```python
from build123d import *

# Parameters (mm, degrees)
F0_R     = 43.18
F1_DEPTH = 330.2
F3_DEPTH = 71.12
F4_R     = 19.05
F5_DEPTH = 76.2
F6_R     = 165.1
F6_R_2   = 19.05
F7_DEPTH = 50.8
F8_R     = 25.39999


# Not quite as in the source:
# - a fillet or chamfer is up to 0.001 mm smaller than in the source, because OpenCascade refuses the exact size


with BuildPart() as f1:
    # F0 (on Top) → F1 (new body)
    with BuildSketch(Plane.XY):
        Circle(F0_R)
    extrude(amount=F1_DEPTH)

    # F2 (on face) → F3 (cut)
    with BuildSketch(Plane(origin=(0, 0, 0), x_dir=(1, 0, 0), z_dir=(0, 0, -1))):
        with BuildLine():
            ThreePointArc((43.18, 0), (40.8909417637, 13.8723927885), (34.2664621733, 26.2739789549))
            Line((34.2664621733, 26.2739789549), (34.2664621733, -26.2739789549))
            ThreePointArc((34.2664621733, -26.2739789549), (40.8909417637, -13.8723927885), (43.18, 0))
        make_face()
    extrude(amount=-F3_DEPTH, mode=Mode.SUBTRACT)

    # F4 (on face) → F5 (join)
    with BuildSketch(Plane.YZ.offset(34.2664621733)):
        with Locations((0, 31.7187957861)):
            Circle(F4_R)
    extrude(amount=F5_DEPTH)

    # F6 (on face) → F7 (join)
    with BuildSketch(Plane.YZ.offset(110.4664621733)):
        with Locations((0, 31.7187957861)):
            Circle(F6_R)
        with Locations((0, 31.7187957861)):
            Circle(F6_R_2, mode=Mode.SUBTRACT)
    extrude(amount=-F7_DEPTH)

    # F8 (radius 25.4 in the source; OpenCascade refuses exactly that, so slightly less here)
    f8_edges = [f1.edges().sort_by_distance(p)[0] for p in [
        (110.466462, -165.1, 31.718796),
        (59.666462, -165.1, 31.718796),
    ]]
    fillet(f8_edges, radius=F8_R)


solid = f1.part
```
Design review of the part built by this model. Coordinates are the model's own, in mm. A direction names the side the tool comes from. Give positions to 0.01 mm unless a question says otherwise; leave off trailing zeros. Loops run counter-clockwise (first coordinate to the right, second up) from the corner with the lowest first, then second, coordinate; pieces in that order, holes last. Notation, with made-up numbers: (52.5, 30) -> (78.5, 30) arc R30 cw to (78.5, 56) -> close; hole circle Ø4 at (14.25, -33). An arc over 180 degrees is marked (long way). One line per item, written item: value.
Q1. We need section D-D on x = 27. Give the boundary of the cut face in (y, z).
Numbers:
outline: (-33.7, 0) -> (33.7, 0) -> (33.7, 330.2) -> (-33.7, 330.2) -> close
Q2. Draft analysis for pull direction X (two halves, no side actions). For faces 4 (the flat face through (-5, 1, 0)), 5 (the flat face through (59.666, -2, 3)), 6 (the flat face through (110.466, -2, 34)), 7 (the cylindrical face through (-43.14, 1.9, 162.79)), state which applies: pulls with the +X half, pulls with the -X half, needs draft (parallel to the pull), parting line crosses it, or undercut.
Numbers:
face 4: needs draft
face 5: undercut
face 6: pulls with the +X half
face 7: undercut
Q3. We need section C-C on z = 225.5. Give the boundary of the cut face in (x, y), and give its area (3 significant figures).
Numbers:
outline: circle Ø86.36 at (0, 0)
area: 5,860 mm^2
Q4. We need section B-B on x = 0. Give the boundary of the cut face in (y, z).
Numbers:
outline: (-43.18, 0) -> (43.18, 0) -> (43.18, 330.2) -> (-43.18, 330.2) -> close
Q5. For L1, parallel to Y at x = -2.5, z = 153; L2, parallel to X at y = 140, z = 30; L3, parallel to Z at x = 16, y = -25, list the stretches that pass through material, from the lowest coordinate up.
Numbers:
L1: y = -43.11 to 43.11
L2: x = 59.67 to 110.46
L3: z = 0 to 330.2
Q6. For pin 1 Ø5 at (y, z) = (-5, 245.5) entering from +X; pin 2 Ø5 at (y, z) = (114, 121) entering from -X; pin 3 Ø2.5 at (x, y) = (39.5, -2) entering from -Z; pin 4 Ø12 at (x, y) = (53.5, -69) entering from -Z, all flat-tipped, find the tip position at first contact; note any pin that passes through.
Numbers:
pin 1: stops at x = 43.11
pin 2: stops at x = 59.8
pin 3: stops at z = 12.68
pin 4: passes through
Q7. Machinability: for faces 1 (the flat face through (38, 0, 71.12)), 2 (the flat face through (-1, 1, 330.2)), 3 (the cylindrical face through (46.79, -15.12, 20.13)), which of the approach directions +Z, -Z, +X, -X, +Y, -Y give a long, thin tool a straight path to every point of the face, cutting with its end or side? Answer none if there is none.
Numbers:
face 1: +Y, -Y
face 2: +Z, +X, -X, +Y, -Y
face 3: none
